Build history of the part. All positions in model axes, mm. A direction names the side the tool comes from. Coordinates: 2 decimals unless noted, no trailing zeros. Write each loop counter-clockwise with the first axis right and the second up, starting at its lowest first coordinate (ties: lowest second). Pieces come first, ordered by that corner, then holes.
```python
from build123d import *

# Parameters (mm, degrees)
BOSS_EXTRUDE1_DEPTH = 11
BOSS_EXTRUDE2_DEPTH = 19.5
SKETCH3_R           = 4
CUT_EXTRUDE1_DEPTH  = 2.5
CUT_EXTRUDE2_DEPTH  = 45
SKETCH5_W           = 44
SKETCH5_H           = 26
BOSS_EXTRUDE3_DEPTH = 5
SKETCH3_3_R         = 4
CUT_EXTRUDE3_DEPTH  = 5


with BuildPart() as part:
    # Sketch1 → Boss-Extrude1 (new body, symmetric)
    with BuildSketch(Plane.XY):
        Polygon((-22, 2.5), (-22, -30), (22, -30), (22, 2.5), (20.5, 2.5), (20.5, -28.5), (-20.5, -28.5), (-20.5, 2.5), align=None)
    extrude(amount=BOSS_EXTRUDE1_DEPTH, both=True)

    # Sketch2 → Boss-Extrude2 (add, symmetric)
    with BuildSketch(Plane(origin=(0, 0, 0), x_dir=(0, 0, -1), z_dir=(1, 0, 0))):
        Polygon((-11, -30), (-13, -30), (-13, -25), (-11.5, -25), (-11.5, -28.5), (-11, -28.5), align=None)
    boss_extrude2 = extrude(amount=BOSS_EXTRUDE2_DEPTH, both=True)

    # Mirror1: Boss-Extrude2 across plane
    add(boss_extrude2.mirror(Plane.XY))

    # Sketch3 → Cut-Extrude1 (cut, through all)
    with BuildSketch(Plane(origin=(0, -28.5, 0), x_dir=(-1, 0, 0), z_dir=(0, 1, 0))):
        Circle(SKETCH3_R)
    extrude(amount=-CUT_EXTRUDE1_DEPTH, mode=Mode.SUBTRACT)

    # Sketch4 → Cut-Extrude2 (cut, through all)
    with BuildSketch(Plane(origin=(22, 0, 0), x_dir=(0, 0, -1), z_dir=(1, 0, 0))):
        with BuildLine():
            Line((-4, 0), (-4, 2.5))
            Line((-4, 2.5), (4, 2.5))
            Line((4, 2.5), (4, 0))
            ThreePointArc((4, 0), (0, -4), (-4, 0))
        make_face()
    extrude(amount=-CUT_EXTRUDE2_DEPTH, mode=Mode.SUBTRACT)

    # Sketch5 → Boss-Extrude3 (add)
    with BuildSketch(Plane.XZ.offset(30)):
        Rectangle(SKETCH5_W, SKETCH5_H)
    extrude(amount=-BOSS_EXTRUDE3_DEPTH)

    # Sketch3<3> → Cut-Extrude3 (cut, symmetric)
    with BuildSketch(Plane(origin=(0, -28.5, 0), x_dir=(-1, 0, 0), z_dir=(0, 1, 0))):
        Circle(SKETCH3_3_R)
    extrude(amount=CUT_EXTRUDE3_DEPTH, both=True, mode=Mode.SUBTRACT)


solid = part.part
```
1. Mould opens along Z. For faces 6 (the face through (0, -28, 13)), 7 (the face through (0, -28, -13)), 8 (the face through (-22, -14, 0)), 9 (the face through (21, 1, -4)) say: +Z half, -Z half, draft (parallel to the pull), parting line (faces both ways), or undercut.
Computed values:
face 6: +Z half
face 7: -Z half
face 8: draft
face 9: undercut
2. 3-axis set-ups, long thin cutter, end or side, ignore diameter. For faces 1 (the face through (-5, -30, 0)), 2 (the face through (-21, 1, 4)), 3 (the face through (20.5, -11, 0)), 4 (the face through (21, -11, 11)), 5 (the face through (-21, -11, -11)): which of +Z, -Z, +X, -X, +Y, -Y reach the whole face in a straight line?
Computed values:
face 1: +Z, -Z, +X, -X, -Y
face 2: +X, -X, +Y
face 3: +Z, -Z, +Y
face 4: +Z, +X, -X, +Y
face 5: -Z, +X, -X, +Y
3. Saw through at A-A on x = 0. List the corners of the cut face in (y, z), plus the area to 3 significant figures.
Computed values:
outline: (-30, -13) - (-25, -13) - (-25, -4) - (-30, -4) - close; (-30, 4) - (-25, 4) - (-25, 13) - (-30, 13) - close
area: 90.0 mm2
4. Saw through at D-D on y = 0.5. List the corners of the cut face in (x, z), plus the area to 3 significant figures.
Computed values:
outline: (-22, -11) - (-20.5, -11) - (-20.5, -4) - (-22, -4) - close; (-22, 4) - (-20.5, 4) - (-20.5, 11) - (-22, 11) - close; (20.5, -11) - (22, -11) - (22, -4) - (20.5, -4) - close; (20.5, 4) - (22, 4) - (22, 11) - (20.5, 11) - close
area: 42.0 mm2
5. Saw through at C-C on y = -11. List the corners of the cut face in (x, z).
Computed values:
outline: (-22, -11) - (-20.5, -11) - (-20.5, 11) - (-22, 11) - close; (20.5, -11) - (22, -11) - (22, 11) - (20.5, 11) - close
6. Probe line 1 along X through (y, z) = (-3.5, -9.5); line 2 along Z through (x, y) = (0, -28); line 3 along Y through (x, z) = (-10.5, 11.25). List the from-to ranges inside material, lowest first.
Computed values:
line 1: x = -22 to -20.5, 20.5 to 22
line 2: z = -13 to -4, 4 to 13
line 3: y = -30 to -25
7. Saw through at B-B on z = 0. List the corners of the cut face in (x, y), plus the area to 3 significant figures.
Computed values:
outline: (-22, -30) - (-4, -30) - (-4, -25) - (-20.5, -25) - (-20.5, -4) - (-22, -4) - close; (4, -30) - (22, -30) - (22, -4) - (20.5, -4) - (20.5, -25) - (4, -25) - close
area: 243 mm2
8. Flat gauge pins, fed straight in: pin 1 (0.8 mm diameter, centred on x = -21, y = -14.5, fed in from +Z); pin 2 (1.2 mm diameter, centred on x = -21.5, y = -9, fed in from -Z); pin 3 (5 mm diameter, centred on x = -1, z = 8.5, fed in from +Y). Where does each tip first touch, or does it go through?
Computed values:
pin 1: stops at z = 11
pin 2: stops at z = -11
pin 3: stops at y = -25
